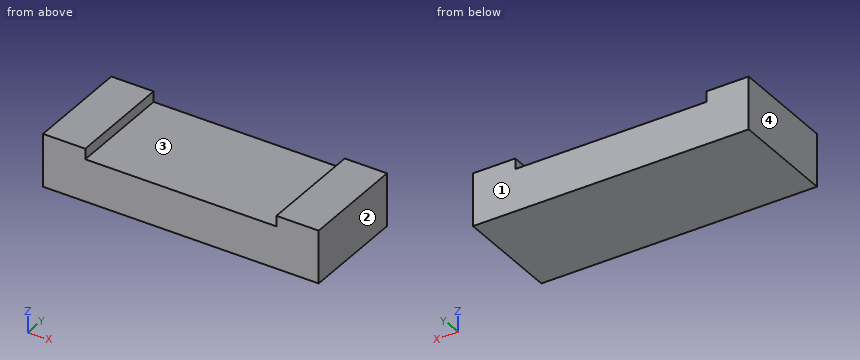
from build123d import *

# Parameters (mm, degrees)
F1_DEPTH = 12.7
F0_W     = 5.842
F0_H     = 12.7
F2_DEPTH = 12.7


with BuildPart() as f1:
    # F0 (on Front) → F1 (new body, symmetric)
    with BuildSketch(Plane.XZ):
        Polygon((5.842, 12.7), (5.842, 0), (66.294, 0), (66.294, 12.7), (56.134, 12.7), (56.134, 10.16), (10.16, 10.16), (10.16, 12.7), align=None)
    extrude(amount=F1_DEPTH, both=True)

    # F0 (on Front) → F2 (join, symmetric)
    with BuildSketch(Plane.XZ):
        with Locations((2.921, 6.35)):
            Rectangle(F0_W, F0_H)
    extrude(amount=F2_DEPTH, both=True)


solid = f1.part
Read the model definition and answer for the solid it produces. Units are mm, in the model's axes. Face numbers are marked on the shaded views. Coordinates: 2 decimals unless noted, no trailing zeros. Loops run counter-clockwise (first coordinate to the right, second up) from the corner with the lowest first, then second, coordinate; pieces in that order, holes last. Notation, with made-up numbers: (-0.75, 77) - (32.25, 77) arc R34 ccw to (32.25, 116) - close; hole circle Ø8 at (34.25, 33.5). An arc over 180 degrees is marked (long way). Answer in a Markdown table with one row per item.
Q1. Find section B-B on y = 10.75. Write down the section's boundary in (x, z).
Here are the results:
| item | result |
|---|---|
| outline | (0, 0) - (66.29, 0) - (66.29, 12.7) - (56.13, 12.7) - (56.13, 10.16) - (10.16, 10.16) - (10.16, 12.7) - (0, 12.7) - close |
Q2. Find section C-C on x = 27.5. Write down the section's boundary in (y, z), plus the area to 3 significant figures.
Here are the results:
| item | result |
|---|---|
| outline | (-12.7, 0) - (12.7, 0) - (12.7, 10.16) - (-12.7, 10.16) - close |
| area | 258 mm^2 |
Q3. Find section A-A on z = 11. Write down the section's boundary in (x, y), plus the area to 3 significant figures.
Here are the results:
| item | result |
|---|---|
| outline | (0, -12.7) - (10.16, -12.7) - (10.16, 12.7) - (0, 12.7) - close; (56.13, -12.7) - (66.29, -12.7) - (66.29, 12.7) - (56.13, 12.7) - close |
| area | 516 mm^2 |
Q4. Given P1, Ø12, axis at x = 34.5, y = 1.5, coming from the +Z side, flat-ended and moving along its own axis, determine where the tip first touches the part or whether it passes through.
Here are the results:
| item | result |
|---|---|
| P1 | stops at z = 10.16 |
Q5. Straight lines are drawn through the part: line 1 along Z through (x, y) = (23.5, 7.25); line 2 along X through (y, z) = (3.5, 10.75). For each, find the intervals that lie inside material, in ascending order. Write a range as [from, to].
Here are the results:
| item | result |
|---|---|
| line 1 | z = [0, 10.16] |
| line 2 | x = [0, 10.16], [56.13, 66.29] |
Q6. The mould has two halves that part along X. Classify the marked faces 1, 2, 3 and 4: pulls with the +X half, pulls with the -X half, needs draft (parallel to the pull), parting line crosses it, or undercut.
Here are the results:
| item | result |
|---|---|
| face 1 | needs draft |
| face 2 | pulls with the +X half |
| face 3 | undercut |
| face 4 | pulls with the -X half |
